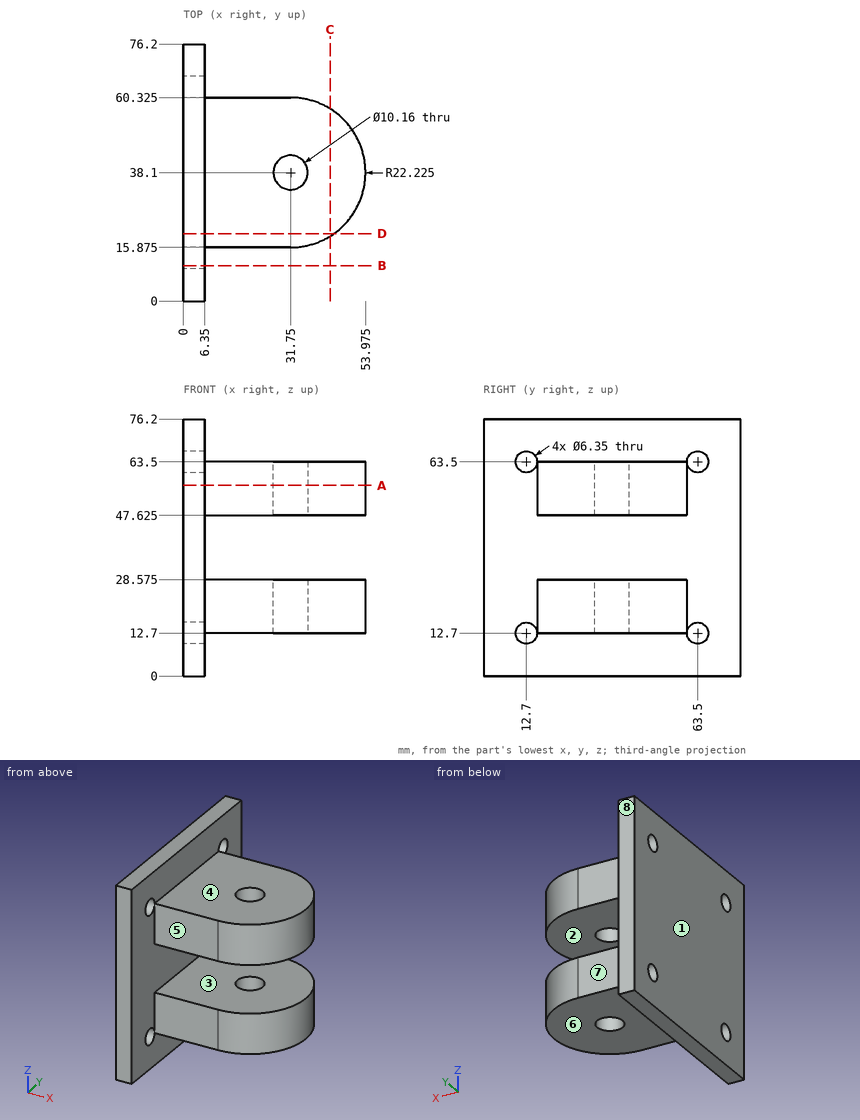
Check sheet for the drawn part. Datum: minimum x, y, z corner. Units: mm. A direction names the side the tool comes from. Round coordinates to 2 decimals unless told otherwise and drop trailing zeros. Loops run counter-clockwise (first coordinate to the right, second up) from the corner with the lowest first, then second, coordinate; pieces in that order, holes last.
Item 1: Mould release check, pull along Z, two halves, no side actions. Record for the marked faces 1, 2, 3 and 4: pulls with the +Z half, pulls with the -Z half, needs draft (parallel to the pull), parting line crosses it, or undercut.
Item 2: Gauge pin test, flat ends, axial feed: pin 1 (22 mm diameter, centred on x = 27, y = 32.5, fed in from -Z); pin 2 (1 mm diameter, centred on x = 47, z = 60, fed in from -Y); pin 3 (12.5 mm diameter, centred on x = 20.5, z = 17.5, fed in from +Y) (3 decimals); pin 4 (4 mm diameter, centred on y = 63.5, z = 63.5, fed in from -X). Record the tip position at first contact, or that the pin passes through.
Item 3: Cross-section at A-A on z = 56.5. Record the boundary of the cut face in (x, y) (3 decimals).
Item 4: Cross-section at B-B on y = 10.5. Record the boundary of the cut face in (x, z).
Item 5: Cross-section at C-C on x = 43.5. Record the boundary of the cut face in (y, z) (3 decimals).
Item 6: Thickness scan on line 1 (Y direction, x = 4, z = 63.5) (3 decimals); line 2 (Z direction, x = 35.5, y = 20) (3 decimals); line 3 (X direction, y = 38, z = 35). Record the ranges inside material, lowest first.
Item 7: Cross-section at D-D on y = 20. Record the boundary of the cut face in (x, z) (3 decimals), then the cut area to 3 significant figures.
Item 8: Access from +Z, -Z, +X, -X, +Y, -Y to the whole of each face (thin tool, end or side, straight path). Record for the marked faces 5, 6, 7 and 8.
Answer sheet:
1. face 1: needs draft
1. face 2: undercut
1. face 3: undercut
1. face 4: pulls with the +Z half
2. pin 1: stops at z = 12.7
2. pin 2: stops at y = 21.48
2. pin 3: stops at y = 60.325
2. pin 4: passes through
3. outline: (0, 0) - (6.35, 0) - (6.35, 15.875) - (31.75, 15.875) arc R22.225 ccw to (31.75, 60.325) - (6.35, 60.325) - (6.35, 76.2) - (0, 76.2) - close; hole circle Ø10.16 at (31.75, 38.1)
4. outline: (0, 0) - (6.35, 0) - (6.35, 10.41) - (0, 10.41) - close; (0, 14.99) - (6.35, 14.99) - (6.35, 61.21) - (0, 61.21) - close; (0, 65.79) - (6.35, 65.79) - (6.35, 76.2) - (0, 76.2) - close
5. outline: (19.235, 12.7) - (56.965, 12.7) - (56.965, 28.575) - (19.235, 28.575) - close; (19.235, 47.625) - (56.965, 47.625) - (56.965, 63.5) - (19.235, 63.5) - close
6. line 1: y = 0 to 9.525, 15.875 to 60.325, 66.675 to 76.2
6. line 2: z = 12.7 to 28.575, 47.625 to 63.5
6. line 3: x = 0 to 6.35
7. outline: (0, 0) - (6.35, 0) - (6.35, 12.7) - (44.647, 12.7) - (44.647, 28.575) - (6.35, 28.575) - (6.35, 47.625) - (44.647, 47.625) - (44.647, 63.5) - (6.35, 63.5) - (6.35, 76.2) - (0, 76.2) - close
7. area: 1,700 mm2
8. face 5: +Z, -Z, +X, -Y
8. face 6: -Z, +X, +Y, -Y
8. face 7: +Z, -Z, +X, +Y
8. face 8: +Z, -Z, +X, -X, +Y
